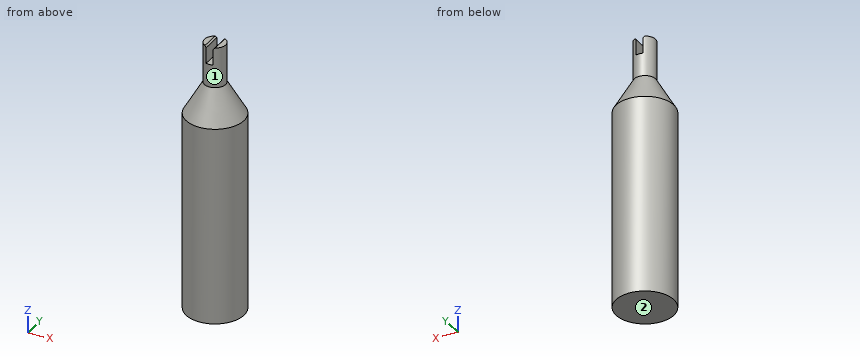
```python
from build123d import *

# Parameters (mm, degrees)
F0_R        = 7.5
F0_R_2      = 2.75
F1_DEPTH    = 60
F2_DEPTH    = 10
F3_S5_R     = 2.75
F3_T6_DEPTH = 13
F5_DEPTH    = 4.5
F6_SIZE     = 0.4


# Not quite as in the source:
# - a fillet or chamfer that OpenCascade refuses, or shapes differently, is made with other operations: its cross-section is extruded or revolved along the edge and cut away or added


with BuildPart() as f1:
    # F0 (on Top) → F1 (new body)
    with BuildSketch(Plane.XY):
        Circle(F0_R)
        Circle(F0_R_2, mode=Mode.SUBTRACT)
        Circle(F0_R_2)
    extrude(amount=-F1_DEPTH)

    # F0 (on Top) → F2 (join)
    with BuildSketch(Plane.XY):
        Circle(F0_R_2)
    extrude(amount=F2_DEPTH)

    # F3: chamfer of 5 x 8.6602540378 on 1 edges, made by hand


with BuildPart() as f3_tool2:
    # F3_s3 → F3_t4 (revolve)
    with BuildSketch(Plane.XZ):
        Polygon((7.5, -8.6602540378), (2.5, 0), (7.5, 0), align=None)
    revolve(axis=Axis((0, 0, 0), (0, 0, 1)))

    # F3_s5 → F3_t6 (cut, symmetric)
    with BuildSketch(Plane.XY.offset(-4.3)):
        Circle(F3_S5_R)
    extrude(amount=F3_T6_DEPTH, both=True, mode=Mode.SUBTRACT)


with BuildPart() as f1_1:
    add(f1.part)

    # F3_t1: cut F3_tool2
    add(f3_tool2.part, mode=Mode.SUBTRACT)

    # F4 (on face) → F5 (cut)
    with BuildSketch(Plane.XY.offset(10)):
        with BuildLine():
            ThreePointArc((-0.9, -2.598557292), (0, -2.75), (0.9, -2.598557292))
            Line((0.9, -2.598557292), (0.9, 2.598557292))
            ThreePointArc((0.9, 2.598557292), (0, 2.75), (-0.9, 2.598557292))
            Line((-0.9, 2.598557292), (-0.9, -2.598557292))
        make_face()
        with BuildLine():
            ThreePointArc((-0.9, 2.598557292), (0, 2.75), (0.9, 2.598557292))
            Line((0.9, 2.598557292), (0.9, 4.5331302099))
            Line((0.9, 4.5331302099), (-0.9, 4.5331302099))
            Line((-0.9, 4.5331302099), (-0.9, 2.598557292))
        make_face()
    extrude(amount=-F5_DEPTH, mode=Mode.SUBTRACT)

    # F6
    f6_edges = [f1_1.edges().sort_by_distance(p)[0] for p in [
        (-0.9, 0, 10),
        (0.9, 0, 10),
    ]]
    chamfer(f6_edges, length=F6_SIZE)


solid = f1_1.part
```
Work out the finished part from the listing and answer in its coordinate system (mm). Face numbers are marked on the shaded views. A direction names the side the tool comes from. Coordinates: 2 decimals unless noted, no trailing zeros. Order: outer loops, then holes, each group sorted by start corner. A loop starts at its lowest first (then second) coordinate and runs counter-clockwise, first axis right, second up. Notation, with made-up numbers: (-17.75, 67) - (-9.75, 67) arc R27 cw to (-9.75, 87) - close; hole circle Ø1 at (-2, 16). An arc over 180 degrees is marked (long way). Answer as a JSON object with one key per item and string values.
1. Find section A-A on y = 0. Determine the outline of the cut face in (x, z), plus the area to 3 significant figures.
Output values:
{"outline": "(-7.5, -60) - (7.5, -60) - (7.5, -8.66) - (2.75, -0.43) - (2.75, 10) - (1.3, 10) - (0.9, 9.6) - (0.9, 5.5) - (-0.9, 5.5) - (-0.9, 9.6) - (-1.3, 10) - (-2.75, 10) - (-2.75, -0.43) - (-7.5, -8.66) - close", "area": "904 mm²"}
2. Find section C-C on z = -18. Determine the outline of the cut face in (x, y), plus the area to 3 significant figures.
Output values:
{"outline": "circle Ø15 at (0, 0)", "area": "177 mm²"}
3. Each of these flat-tipped pins is pushed along its axis until it touches: P1, Ø1.4, axis at x = -0.5, y = 0.5, coming from the +Z side; P2, Ø1, axis at y = -2.5, z = -10, coming from the +X side; P3, Ø1, axis at y = -5, z = -8.5, coming from the +X side. Where does it stop, or does it pass through?
Output values:
{"P1": "stops at z = 9.9", "P2": "stops at x = 7.23", "P3": "stops at x = 5.98"}
4. A tool of negligible diameter and unlimited length cuts with its end or side. For the marked faces 1 and 2, from which of +Z, -Z, +X, -X, +Y, -Y can it reach the whole face along a straight path? Write none if from no direction.
Output values:
{"face 1": "+Z", "face 2": "-Z, +X, -X, +Y, -Y"}
5. Consider line 1 (Z direction, x = 3.25, y = -6); line 2 (Z direction, x = 0.5, y = -2); line 3 (Y direction, x = -0.25, z = -34). Determine where each line is inside the solid, lowest interval first.
Output values:
{"line 1": "z = -60 to -7.49", "line 2": "z = -60 to 5.5", "line 3": "y = -7.5 to 7.5"}
6. Find section B-B on x = 0. Determine the outline of the cut face in (y, z), plus the area to 3 significant figures.
Output values:
{"outline": "(-7.5, -60) - (7.5, -60) - (7.5, -8.66) - (2.75, -0.43) - (2.75, 5.5) - (-2.75, 5.5) - (-2.75, -0.43) - (-7.5, -8.66) - close", "area": "887 mm²"}
